Autodesk Inventor part; units mm, degrees
ref_plane "YZ Plane" through (0, 0, 0) normal (1, 0, 0) x (0, 1, 0)
ref_plane "XZ Plane" through (0, 0, 0) normal (0, 1, 0) x (-1, 0, 0)
ref_plane "XY Plane" through (0, 0, 0) normal (0, 0, 1) x (1, 0, 0)
sketch "Sketch1" plane through (0, 0, 0) normal (0, 1, 0) x (-1, 0, 0)
  circle A0 centre (0, 0) radius 9.75
  circle A1 centre (0, 0) radius 12.75
  dimension "d0" = 19.5
  dimension "d1" = 3
extrude "Extrusion1" add sketch "Sketch1" along normal blind 100
sketch "Sketch2" plane through (0, 0, 0) normal (0, -1, 0) x (1, 0, 0)
  circle A0 centre (0, 0) radius 5
  circle A1 centre (0, 0) radius 7
  dimension "d4" = 10
  dimension "d5" = 14
extrude "Extrusion2" add sketch "Sketch2" against normal blind 2
sketch "Sketch3" plane through (0, 0, 0) normal (0, -1, 0) x (1, 0, 0)
  circle A0 centre (0, 0) radius 12.75
extrude "Extrusion3" add sketch "Sketch3" along normal blind 5
sketch "Sketch4" plane through (0, -5, 0) normal (0, -1, 0) x (1, 0, 0)
  circle A0 centre (0, 0) radius 25
  circle A1 centre (0, 0) radius 7
  circle A2 centre (0, 0) radius 20
  circle A3 centre (-20, 0) radius 3
  circle A4 centre (0, 20) radius 3
  circle A5 centre (20, 0) radius 3
  circle A6 centre (0, -20) radius 3
  circle A7 centre (0, 0) radius 12.75
  line L0 (-20, 0) -> (0, 0)
  circle A8 centre (0, 0) radius 9.75
  line L1 (0, 20) -> (0, 0)
  circle A9 centre (0, 0) radius 5
  line L2 (20, 0) -> (0, 0)
  line L3 (0, -20) -> (0, 0)
  circle A10 centre (14.1421, -14.1421) radius 3
  line L4 (14.1421, -14.1421) -> (0, 0)
  line L5 (-35, 0) -> (35, 0)
  dimension "d10" = 50
  dimension "d11" = 40
  dimension "d12" = 90
  dimension "d13" = 90
  dimension "d14" = 90
  dimension "d15" = 45
  dimension "d16" = 6
extrude "Extrusion4" add sketch "Sketch4" against normal blind 5 contours L5 A5 A2 A4 A3 A0 | A0 L5 A3 A2 A6 A10 A5 | A5 L2 A7 L1 A4 A2 | A2 A10 L4 A7 L2 A5 | A2 A4 L1 A7 L0 A3 | A3 L0 A7 L3 A6 A2 | L2 A8 L1 A7 | A7 L4 A8 L2 | A10 A2 A6 L3 A7 L4 | L0 A8 L3 A7 | A7 L1 A8 L0 | A7 L3 A8 L4 | L2 A1 L1 A8 | A8 L4 A1 L2 | A8 L1 A1 L0 | L0 A1 L3 A8 | A8 L3 A1 L4 | L2 A9 L1 A1 | A1 L4 A9 L2 | L0 A9 L3 A1 | A1 L1 A9 L0 | A1 L3 A9 L4 | L2 L1 A9 | A9 L4 L2 | A9 L1 L0 | L0 L3 A9 | A9 L3 L4
sketch "Sketch5" plane through (0, 100, 0) normal (0, 1, 0) x (1, 0, 0)
  circle A0 centre (0, 0) radius 12.75
  circle A1 centre (0, 0) radius 9.75
  line L0 (1.9927, -8.75) -> (-2.0073, -8.75)
  line L1 (-2.0073, -8.75) -> (-2.0073, -16.75)
  line L2 (-2.0073, -16.75) -> (1.9927, -16.75)
  line L3 (1.9927, -16.75) -> (1.9927, -8.75)
  circle A2 centre (0, 0) radius 12.75
  line L4 (1.9927, -8.75) -> (-2.0073, -16.75) construction
  line L5 (-2.0073, -8.75) -> (1.9927, -16.75) construction
  line L6 (1.9927, 8.75) -> (-2.0073, 8.75)
  line L7 (-2.0073, 8.75) -> (-2.0073, 16.75)
  line L8 (-2.0073, 16.75) -> (1.9927, 16.75)
  line L9 (1.9927, 16.75) -> (1.9927, 8.75)
  line L10 (1.9927, 8.75) -> (-2.0073, 16.75) construction
  line L11 (-2.0073, 8.75) -> (1.9927, 16.75) construction
  point P0 (-0.0073, -12.75)
  point P1 (-0.0073, 12.75)
  point P2 (1.9927, -12.5933)
  point P3 (-2.0073, -12.591)
  point P4 (-2.0073, 12.591)
  point P5 (1.9927, 12.5933)
  dimension "d19" = 4
  dimension "d20" = 8
extrude "Extrusion5" add sketch "Sketch5" against normal blind 4 contours A0 L7 L8 L9 | L3 L2 L1 A0
properties part number "Base"
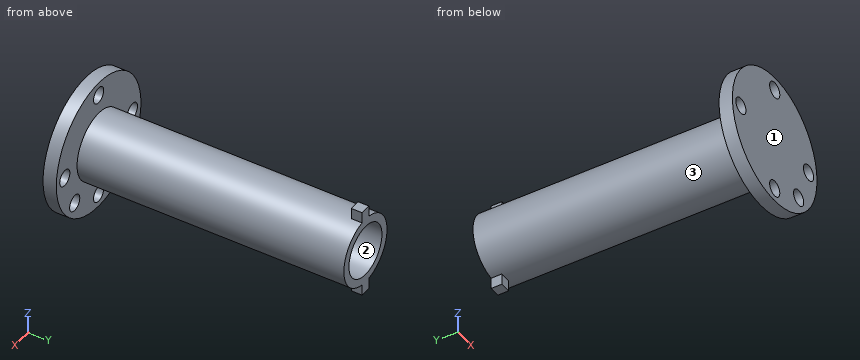
The model under review builds one solid part; all positions refer to its coordinate system, in mm. Face numbers are marked on the shaded views. Round coordinates to 2 decimals unless told otherwise and drop trailing zeros. Write each loop counter-clockwise with the first axis right and the second up, starting at its lowest first coordinate (ties: lowest second). Pieces come first, ordered by that corner, then holes. Notation, with made-up numbers: (21.25, 37) -> (49.25, 37) arc R21 cw to (49.25, 42) -> close; hole circle Ø8 at (63, -22). An arc over 180 degrees is marked (long way). Answer as a JSON object with one key per item and string values.
1. To check wall thickness, follow line 1 along Z through (x, y) = (0, -4); line 2 along Z through (x, y) = (0, 9.5). State the ranges of each line that lie inside material, in increasing order.
Results found:
{"line 1": "z = -25 to -23, -17 to 17, 23 to 25", "line 2": "z = -12.75 to -9.75, 9.75 to 12.75"}
2. The part is to be moulded in two halves that separate along X. For the marked faces 1, 2 and 3, say which applies: pulls with the +X half, pulls with the -X half, needs draft (parallel to the pull), parting line crosses it, or undercut.
Results found:
{"face 1": "needs draft", "face 2": "undercut", "face 3": "parting line crosses it"}
3. We need section C-C on z = 15. State the section outline as (x, y) points, and give its area (3 significant figures).
Results found:
{"outline": "(-20, -5) -> (20, -5) -> (20, 0) -> (-20, 0) -> close; (-2.01, 96) -> (1.99, 96) -> (1.99, 100) -> (-2.01, 100) -> close", "area": "216 mm^2"}
4. We need section D-D on x = -20. State the section outline as (y, z) points, and give its area (3 significant figures).
Results found:
{"outline": "(-5, -15) -> (0, -15) -> (0, -3) -> (-5, -3) -> close; (-5, 3) -> (0, 3) -> (0, 15) -> (-5, 15) -> close", "area": "120 mm^2"}
5. We need section A-A on z = 0. State the section outline as (x, y) points.
Results found:
{"outline": "(-25, -5) -> (-23, -5) -> (-23, 0) -> (-25, 0) -> close; (-17, -5) -> (17, -5) -> (17, 0) -> (12.75, 0) -> (12.75, 100) -> (9.75, 100) -> (9.75, 0) -> (7, 0) -> (7, 2) -> (5, 2) -> (5, 0) -> (-5, 0) -> (-5, 2) -> (-7, 2) -> (-7, 0) -> (-9.75, 0) -> (-9.75, 100) -> (-12.75, 100) -> (-12.75, 0) -> (-17, 0) -> close; (23, -5) -> (25, -5) -> (25, 0) -> (23, 0) -> close"}
6. We need section B-B on x = 0. State how many separate pieces and enclosed holes the cut face has, and give its area (3 significant figures).
Results found:
{"separate pieces": "3", "enclosed holes": "0", "area": "830 mm^2"}
7. Clearance check with flat-ended pins moving along their axes: pin 1 (25 mm diameter, centred on x = 5.5, z = -4.5, fed in from +Y); pin 2 (11.5 mm diameter, centred on x = 0, z = 0, fed in from +Y); pin 3 (3 mm diameter, centred on x = 0, y = 98.5, fed in from +Z); pin 4 (9.5 mm diameter, centred on x = 20, z = 0, fed in from +Y). State where each tip first meets the part, or that it passes through.
Results found:
{"pin 1": "stops at y = 100", "pin 2": "stops at y = 2", "pin 3": "stops at z = 16.75", "pin 4": "stops at y = 0"}
